```python
from build123d import *

# Parameters (mm, degrees)
SKETCH1_W           = 483
SKETCH1_H           = 135
BOSS_EXTRUDE1_DEPTH = 610
SKETCH2_W           = 17
SKETCH2_H           = 135
CUT_EXTRUDE1_DEPTH  = 605
SKETCH4_R           = 5


with BuildPart() as part:
    # Sketch1 → Boss-Extrude1 (new body)
    with BuildSketch(Plane.XY):
        with Locations((241.5, 67.5)):
            Rectangle(SKETCH1_W, SKETCH1_H)
    extrude(amount=-BOSS_EXTRUDE1_DEPTH)

    # Sketch2 → Cut-Extrude1 (cut)
    with BuildSketch(Plane(origin=(0, 0, -610), x_dir=(-1, 0, 0), z_dir=(0, 0, -1))):
        with Locations((-474.5, 67.5)):
            Rectangle(SKETCH2_W, SKETCH2_H)
        with Locations((-8.5, 67.5)):
            Rectangle(SKETCH2_W, SKETCH2_H)
    extrude(amount=-CUT_EXTRUDE1_DEPTH, mode=Mode.SUBTRACT)

    # Sweep1: sweep along a path in Sketch3
    with BuildLine(Plane(origin=(460, 0, 0), x_dir=(0, 0, -1), z_dir=(1, 0, 0))) as sweep1_path:
        Line((0, 117.5), (-30, 117.5))
        ThreePointArc((-30, 117.5), (-37.071067812, 114.571067812), (-40, 107.5))
        Line((-40, 107.5), (-40, 27.5))
        ThreePointArc((-40, 27.5), (-37.071067812, 20.428932188), (-30, 17.5))
        Line((-30, 17.5), (0, 17.5))
    # Sketch4 → Sweep1 (sweep)
    with BuildSketch(Plane.XY):
        with Locations((460, 117.5)):
            Circle(SKETCH4_R)
    sweep1 = sweep(path=sweep1_path.line)

    # Mirror1: Sweep1 across plane
    add(sweep1.mirror(Plane(origin=(241.5, 0, 0), x_dir=(0, 0, 1), z_dir=(1, 0, 0))))


solid = part.part
```
Here's how the part is built. I have some questions about the finished solid (model axes, mm). A direction names the side the tool comes from. Give positions to 0.01 mm unless a question says otherwise; leave off trailing zeros. Order: outer loops, then holes, each group sorted by start corner. A loop starts at its lowest first (then second) coordinate and runs counter-clockwise, first axis right, second up. Notation, with made-up numbers: (23, 43) - (33, 43) arc R24 cw to (33, 61) - close; hole circle Ø2 at (-4, -0.75). An arc over 180 degrees is marked (long way). Answer as a JSON object with one key per item and string values. Group by question number.
Item 1: If we section it at A-A on y = 90.5: Please give me the cut outline in (x, z), and give its area (3 significant figures).
Item 2: For P1, Ø12, axis at x = 58, y = 107.5, coming from the +Z side; P2, Ø8, axis at y = 91.5, z = -80.5, coming from the -X side; P3, Ø4, axis at y = 18.5, z = -149.5, coming from the +X side, each with a flat end and sliding along its axis, tell me the tip position at first contact or that it passes through.
Item 3: If we section it at C-C on x = 350: Please give me the cut outline in (y, z), and give its area (4 significant figures).
Item 4: If we section it at B-B on z = -360: Please give me the cut outline in (x, y), and give its area (3 significant figures).
Item 5: If we mould it in two halves opening along Z, with no side actions, what happens to faces 4 (the flat face through (238, 68, -610)), 5 (the flat face through (17, 67, -312))? For each: pulls with the +Z half, pulls with the -Z half, needs draft (parallel to the pull), parting line crosses it, or undercut.
Item 6: Which directions (+Z, -Z, +X, -X, +Y, -Y) give clear straight access to the entire face, cutting with the end or side of a thin tool? Please do faces 1 (the flat face through (238, 0, -301)), 2 (the flat face through (466, 67, -312)), 3 (the flat face through (9, 68, -5)).
Item 7: Please list where these lines run through material, in increasing order: probe 1 along X at (y, z) = (12, -193); probe 2 along Z at (x, y) = (137, 23); probe 3 along Z at (x, y) = (20, 70).
Result set:
{
 "1": {"outline": "(0, -5) - (17, -5) - (17, -610) - (466, -610) - (466, -5) - (483, -5) - (483, 0) - (0, 0) - close; circle Ø10 at (23, 40); circle Ø10 at (460, 40)", "area": "274,000 mm²"},
 "2": {"P1": "z = 0", "P2": "x = 17", "P3": "x = 466"},
 "3": {"outline": "(0, -610) - (135, -610) - (135, 0) - (0, 0) - close", "area": "82,350 mm²"},
 "4": {"outline": "(17, 0) - (466, 0) - (466, 135) - (17, 135) - close", "area": "60,600 mm²"},
 "5": {"face 4": "pulls with the -Z half", "face 5": "needs draft"},
 "6": {"face 1": "+Z, -Z, +X, -X, -Y", "face 2": "-Z, +X, +Y, -Y", "face 3": "-Z, -X, +Y, -Y"},
 "7": {"probe 1": "17 to 466", "probe 2": "-610 to 0", "probe 3": "-610 to 0, 36 to 44"}
}
